Could you check a few things on this model? Use its own coordinates, in mm. Round coordinates to 2 decimals unless told otherwise and drop trailing zeros. Write each loop counter-clockwise with the first axis right and the second up, starting at its lowest first coordinate (ties: lowest second). Pieces come first, ordered by that corner, then holes. Notation, with made-up numbers: (-2.5, 2.5) -> (11.5, 2.5) arc R26 cw to (11.5, 34.5) -> close; hole circle Ø4 at (36, -10). An arc over 180 degrees is marked (long way). Return JSON: item names as keys, results as strings.
from build123d import *

# Parameters (mm, degrees)
BOSS_EXTRUDE1_DEPTH = 23.8125
SKETCH2_W           = 3.175
SKETCH2_H           = 25.4
SKETCH2_H_2         = 22.557316078
CUT_EXTRUDE1_DEPTH  = 3.175


with BuildPart() as part:
    # Sketch1 → Boss-Extrude1 (new body)
    with BuildSketch(Plane.XY):
        Polygon((322.665849031, 315.38832698), (306.887039832, 270.101095383), (309.885267674, 269.056463963), (325.664076873, 314.34369556), align=None)
    extrude(amount=-BOSS_EXTRUDE1_DEPTH)

    # Sketch2 → Cut-Extrude1 (cut)
    with BuildSketch(Plane(origin=(192.743701136, -67.155045192, 0), x_dir=(0, 0, -1), z_dir=(0.94432373, -0.32901777, 0))):
        with Locations((22.225, 391.291479466)):
            Rectangle(SKETCH2_W, SKETCH2_H)
        with Locations((1.5875, 380.012821427)):
            Rectangle(SKETCH2_W, SKETCH2_H_2)
    extrude(amount=-CUT_EXTRUDE1_DEPTH, mode=Mode.SUBTRACT)


solid = part.part
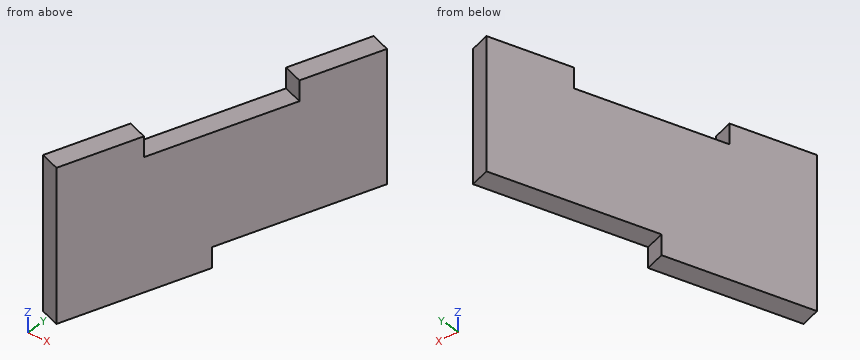
1) I want a section at C-C, the plane y = 276. Please give me the cut outline in (x, z), and give its area (3 significant figures).
Return value:
{"outline": "(308.94, -23.81) -> (312.3, -23.81) -> (312.3, 0) -> (308.94, 0) -> close", "area": "80.1 mm²"}
2) Will these pins go through, and if not, where does the flat tip stop? pin 1 Ø5.5 at (x, y) = (318.5, 299.5) entering from -Z; pin 2 Ø3 at (x, y) = (315, 297.5) entering from +Z (3 decimals); pin 3 Ø8 at (y, z) = (283.5, -8) entering from +X.
Return value:
{"pin 1": "z = -20.64", "pin 2": "z = -3.175", "pin 3": "x = 316.31"}
3) I want a section at B-B, the plane z = -15. Please give me the cut outline in (x, y).
Return value:
{"outline": "(306.89, 270.1) -> (309.89, 269.06) -> (325.66, 314.34) -> (322.67, 315.39) -> close"}
4) I want a section at A-A, the plane x = 319.5. Please give me the cut outline in (y, z) (1 decimal).
Return value:
{"outline": "(296.7, -20.6) -> (306.3, -20.6) -> (306.3, 0) -> (303, 0) -> (303, -3.2) -> (296.7, -3.2) -> close"}
5) If I drill on probe 1 along Z at (x, y) = (318.5, 296) (1 decimal); probe 2 along X at (y, z) = (283, -17.5); probe 3 along X at (y, z) = (272, -1.25), over which ranges is the centre line in solid material (lowest first)? Write a range as [from, to].
Return value:
{"probe 1": "[-20.6, -3.2]", "probe 2": "[311.38, 314.74]", "probe 3": "[307.55, 310.91]"}
